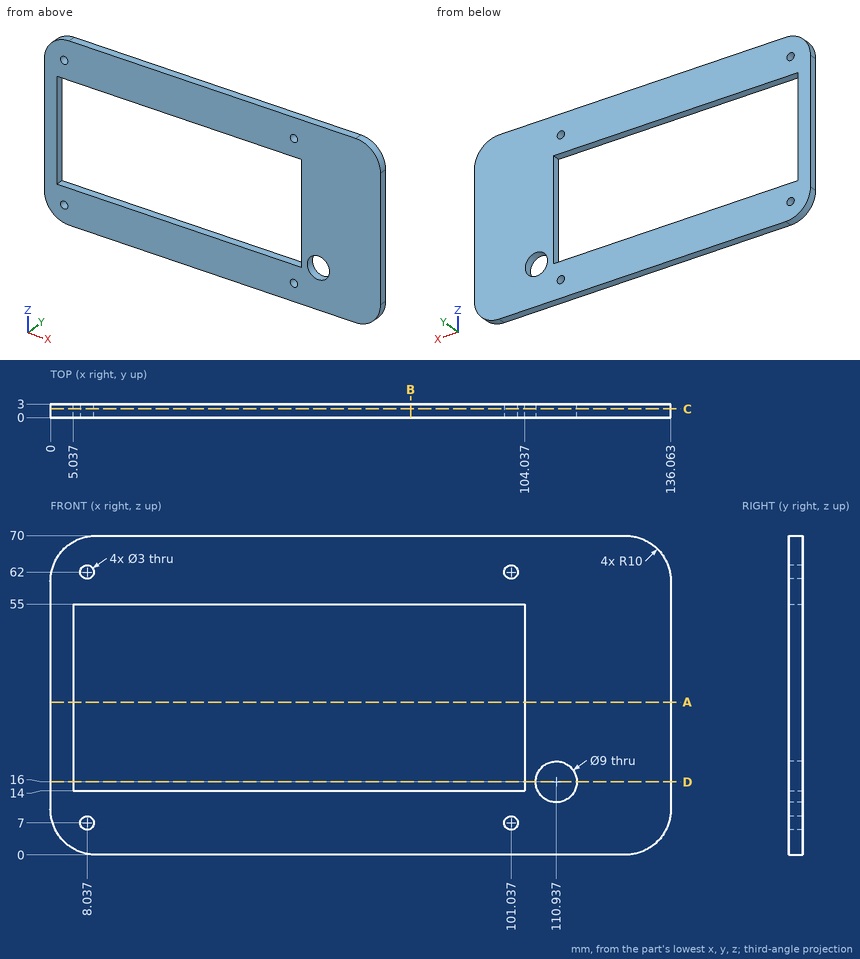
Source: three-view drawing plus pictorial views. Frame: mm from the lowest corner of the part. Round coordinates to 2 decimals unless told otherwise and drop trailing zeros. Loops run counter-clockwise (first coordinate to the right, second up) from the corner with the lowest first, then second, coordinate; pieces in that order, holes last.
1. Ray query, L1, parallel to Z at x = 18.5, y = 2.5; L2, parallel to X at y = 1.45, z = 6 (1 decimal); L3, parallel to X at y = 1.45, z = 27.5. Return the intervals inside material, ascending.
2. Section query D-D on z = 16. Output: boundary loops of the cut face in (x, y).
3. Section query C-C on y = 1.95. Output: boundary loops of the cut face in (x, z), and give its area (3 significant figures).
4. Section query A-A on z = 33.5. Output: boundary loops of the cut face in (x, y).
5. Section query B-B on x = 79. Output: boundary loops of the cut face in (y, z).
6. Contact query for a flat-ended pin moving along its axis: pin 1 (3.5 mm diameter, centred on x = 8.04, z = 62, fed in from -Y). Output: stop coordinate, or through.
Answers below:
1. L1: z = 0 to 14, 55 to 70
1. L2: x = 0.8 to 6.9, 9.2 to 99.9, 102.2 to 135.2
1. L3: x = 0 to 5.04, 104.04 to 136.06
2. outline: (0, 0) - (5.04, 0) - (5.04, 3) - (0, 3) - close; (104.04, 0) - (106.44, 0) - (106.44, 3) - (104.04, 3) - close; (115.44, 0) - (136.06, 0) - (136.06, 3) - (115.44, 3) - close
3. outline: (0, 10) arc R10 ccw to (10, 0) - (126.06, 0) arc R10 ccw to (136.06, 10) - (136.06, 60) arc R10 ccw to (126.06, 70) - (10, 70) arc R10 ccw to (0, 60) - close; hole (5.04, 14) - (104.04, 14) - (104.04, 55) - (5.04, 55) - close; hole circle Ø3 at (8.04, 7); hole circle Ø3 at (8.04, 62); hole circle Ø3 at (101.04, 7); hole circle Ø3 at (101.04, 62); hole circle Ø9 at (110.94, 16)
3. area: 5,290 mm2
4. outline: (0, 0) - (5.04, 0) - (5.04, 3) - (0, 3) - close; (104.04, 0) - (136.06, 0) - (136.06, 3) - (104.04, 3) - close
5. outline: (0, 0) - (3, 0) - (3, 14) - (0, 14) - close; (0, 55) - (3, 55) - (3, 70) - (0, 70) - close
6. pin 1: stops at y = 0
